Input: part model. Units: mm. Frame: model coordinates. A direction names the side the tool comes from. Round coordinates to 2 decimals unless told otherwise and drop trailing zeros. Order: outer loops, then holes, each group sorted by start corner. A loop starts at its lowest first (then second) coordinate and runs counter-clockwise, first axis right, second up. Notation, with made-up numbers: (-22, 43) - (1, 43) arc R6 cw to (1, 52) - close; hole circle Ø1 at (88, -16.5). An arc over 180 degrees is marked (long way). One line per item, written item: value. Start each with the question number.
from build123d import *

# Parameters (mm, degrees)
SKETCH1_W           = 31
SKETCH1_H           = 15
BOSS_EXTRUDE1_DEPTH = 6
SKETCH2_W           = 20.15
SKETCH2_H           = 6.15
CUT_EXTRUDE1_DEPTH  = 13
SKETCH6_R           = 5.45
SKETCH6_R_2         = 2.95
BOSS_EXTRUDE3_DEPTH = 3
CUT_EXTRUDE3_REACH  = 24.035
SKETCH3_W           = 1
SKETCH3_H           = 4
SKETCH3_W_2         = 2
SKETCH3_H_2         = 3.5
CUT_EXTRUDE4_START  = -3
SKETCH7_W           = 0.511909323
SKETCH7_H           = 0.870011062
SKETCH7_W_2         = 0.855337353
SKETCH7_H_2         = 1.408005392
CUT_EXTRUDE4_DEPTH  = 3
SKETCH8_W           = 31
SKETCH8_H           = 12
CUT_EXTRUDE5_DEPTH  = 3
CUT_EXTRUDE6_REACH  = 25.126
SKETCH9_R           = 1
SKETCH10_R          = 2.625
CUT_EXTRUDE7_DEPTH  = 2
SKETCH11_R          = 2.625
CUT_EXTRUDE8_DEPTH  = 2
CUT_EXTRUDE9_DEPTH  = 15
FILLET3_R           = 0.75
CUT_EXTRUDE10_DEPTH = 12
CHAMFER2_SIZE       = 1
FILLET4_R           = 0.75
CHAMFER3_SIZE       = 1.25
CUT_EXTRUDE11_DEPTH = 0.4


with BuildPart() as part:
    # Sketch1 → Boss-Extrude1 (new, symmetric)
    with BuildSketch(Plane.XY):
        Rectangle(SKETCH1_W, SKETCH1_H)
    extrude(amount=BOSS_EXTRUDE1_DEPTH, both=True)

    # Sketch2 → Cut-Extrude1 (cut)
    with BuildSketch(Plane.XZ.offset(7.5)):
        Rectangle(SKETCH2_W, SKETCH2_H)
    extrude(amount=-CUT_EXTRUDE1_DEPTH, mode=Mode.SUBTRACT)

    # Sketch6 → Boss-Extrude3 (add)
    # profile 1 of 2: a face of its own
    with BuildSketch(Plane(origin=(0, 7.5, 0), x_dir=(1, 0, 0), z_dir=(0, 1, 0))):
        with Locations(Location((-11.3, 0, 0), (0, 0, 140.41159309))):
            Circle(SKETCH6_R)
        with Locations(Location((-11.3, 0, 0), (0, 0, 270))):
            Circle(SKETCH6_R_2, mode=Mode.SUBTRACT)
    # profile 2 of 2: a face of its own
    with BuildSketch(Plane(origin=(0, 7.5, 0), x_dir=(1, 0, 0), z_dir=(0, 1, 0))):
        with Locations(Location((11.3, 0, 0), (0, 0, 39.58840691))):
            Circle(SKETCH6_R)
        with Locations(Location((11.3, 0, 0), (0, 0, 270))):
            Circle(SKETCH6_R_2, mode=Mode.SUBTRACT)
    extrude(amount=BOSS_EXTRUDE3_DEPTH)

    # Cut-Extrude3: up to this face of the body (flat: up to its plane)
    cut_extrude3_end = Plane(part.part.faces().sort_by_distance((-7.218793939, 10.5, 3.374876584))[0])
    # Sketch3 → Cut-Extrude3 (cut, up to the picked face)
    with BuildSketch(Plane.XZ.offset(-5.5), mode=Mode.PRIVATE) as cut_extrude3_sk1:
        with Locations((8.075, 0)):
            Rectangle(SKETCH3_W, SKETCH3_H)
    cut_extrude3_tool1 = split(extrude(cut_extrude3_sk1.sketch, amount=-CUT_EXTRUDE3_REACH, mode=Mode.PRIVATE), bisect_by=cut_extrude3_end, keep=Keep.BOTH, mode=Mode.PRIVATE)
    # Sketch3 → Cut-Extrude3 (cut, up to the picked face)
    with BuildSketch(Plane.XZ.offset(-5.5), mode=Mode.PRIVATE) as cut_extrude3_sk2:
        with Locations((-8.075, 0)):
            Rectangle(SKETCH3_W, SKETCH3_H)
    cut_extrude3_tool2 = split(extrude(cut_extrude3_sk2.sketch, amount=-CUT_EXTRUDE3_REACH, mode=Mode.PRIVATE), bisect_by=cut_extrude3_end, keep=Keep.BOTH, mode=Mode.PRIVATE)
    # Sketch3 → Cut-Extrude3 (cut, up to the picked face)
    with BuildSketch(Plane.XZ.offset(-5.5), mode=Mode.PRIVATE) as cut_extrude3_sk3:
        with Locations((-0.825, 0)):
            Rectangle(SKETCH3_W_2, SKETCH3_H_2)
    cut_extrude3_tool3 = split(extrude(cut_extrude3_sk3.sketch, amount=-CUT_EXTRUDE3_REACH, mode=Mode.PRIVATE), bisect_by=cut_extrude3_end, keep=Keep.BOTH, mode=Mode.PRIVATE)
    add(cut_extrude3_tool1.solids().sort_by(Axis((8.075, 5.5, 0), (0, 1, 0)))[0], mode=Mode.SUBTRACT)
    add(cut_extrude3_tool2.solids().sort_by(Axis((-8.075, 5.5, 0), (0, 1, 0)))[0], mode=Mode.SUBTRACT)
    add(cut_extrude3_tool3.solids().sort_by(Axis((-0.825, 5.5, 0), (0, 1, 0)))[0], mode=Mode.SUBTRACT)

    # Sketch7 → Cut-Extrude4 (cut)
    with BuildSketch(Plane(origin=(0, 10.5, 0), x_dir=(1, 0, 0), z_dir=(0, 1, 0)).offset(CUT_EXTRUDE4_START)):
        with BuildLine():
            ThreePointArc((-8.575, 1.129988938), (-8.814868985, 1.58953573), (-9.131475156, 2))
            Line((-9.131475156, 2), (-9.143163494, 2))
            Line((-9.143163494, 2), (-9.143163494, 0.699379733))
            Line((-9.143163494, 0.699379733), (-8.575, 0.699379733))
            Line((-8.575, 0.699379733), (-8.575, 1.129988938))
        make_face()
        with BuildLine():
            Line((-8.575, 1.129988938), (-8.575, 2))
            Line((-8.575, 2), (-9.131475156, 2))
            ThreePointArc((-9.131475156, 2), (-8.814868985, 1.58953573), (-8.575, 1.129988938))
        make_face()
        with BuildLine():
            ThreePointArc((-8.575, -1.129988938), (-8.814868985, -1.58953573), (-9.131475156, -2))
            Line((-9.131475156, -2), (-8.575, -2))
            Line((-8.575, -2), (-8.575, -1.129988938))
        make_face()
        with BuildLine():
            Line((-9.143163494, -2), (-9.131475156, -2))
            ThreePointArc((-9.131475156, -2), (-8.814868985, -1.58953573), (-8.575, -1.129988938))
            Line((-8.575, -1.129988938), (-8.575, -0.709964508))
            Line((-8.575, -0.709964508), (-9.143163494, -0.709964508))
            Line((-9.143163494, -0.709964508), (-9.143163494, -2))
        make_face()
        with Locations((8.830954662, 1.564994469)):
            Rectangle(SKETCH7_W, SKETCH7_H)
        with Locations((9.002668677, -1.295997304)):
            Rectangle(SKETCH7_W_2, SKETCH7_H_2)
    extrude(amount=CUT_EXTRUDE4_DEPTH, mode=Mode.SUBTRACT)

    # Sketch8 → Cut-Extrude5 (cut)
    with BuildSketch(Plane.XZ.offset(7.5)):
        Rectangle(SKETCH8_W, SKETCH8_H)
    extrude(amount=-CUT_EXTRUDE5_DEPTH, mode=Mode.SUBTRACT)

    # Cut-Extrude6: up to this face of the body (flat: up to its plane)
    cut_extrude6_end = Plane(part.part.faces().sort_by_distance((0, 1.5, -6))[0])
    # Sketch9 → Cut-Extrude6 (cut, up to the picked face)
    with BuildSketch(Plane.XY.offset(6), mode=Mode.PRIVATE) as cut_extrude6_sk1:
        with Locations((4.82, 1.5)):
            Circle(SKETCH9_R)
    cut_extrude6_tool1 = split(extrude(cut_extrude6_sk1.sketch, amount=-CUT_EXTRUDE6_REACH, mode=Mode.PRIVATE), bisect_by=cut_extrude6_end, keep=Keep.BOTH, mode=Mode.PRIVATE)
    # Sketch9 → Cut-Extrude6 (cut, up to the picked face)
    with BuildSketch(Plane.XY.offset(6), mode=Mode.PRIVATE) as cut_extrude6_sk2:
        with Locations((-4.82, 1.5)):
            Circle(SKETCH9_R)
    cut_extrude6_tool2 = split(extrude(cut_extrude6_sk2.sketch, amount=-CUT_EXTRUDE6_REACH, mode=Mode.PRIVATE), bisect_by=cut_extrude6_end, keep=Keep.BOTH, mode=Mode.PRIVATE)
    add(cut_extrude6_tool1.solids().sort_by(Axis((4.82, 1.5, 6), (0, 0, -1)))[0], mode=Mode.SUBTRACT)
    add(cut_extrude6_tool2.solids().sort_by(Axis((-4.82, 1.5, 6), (0, 0, -1)))[0], mode=Mode.SUBTRACT)

    # Sketch10 → Cut-Extrude7 (cut)
    with BuildSketch(Plane.XY.offset(6)):
        with Locations((4.82, 1.5)):
            Circle(SKETCH10_R)
    extrude(amount=-CUT_EXTRUDE7_DEPTH, mode=Mode.SUBTRACT)

    # Sketch11 → Cut-Extrude8 (cut)
    with BuildSketch(Plane(origin=(0, 0, -6), x_dir=(-1, 0, 0), z_dir=(0, 0, -1))):
        with Locations((4.82, 1.5)):
            Circle(SKETCH11_R)
    extrude(amount=-CUT_EXTRUDE8_DEPTH, mode=Mode.SUBTRACT)

    # Sketch12 → Cut-Extrude9 (cut)
    with BuildSketch(Plane.XZ.offset(4.5)):
        with BuildLine():
            Line((15.5, 3.473110997), (15.5, -3.473110997))
            ThreePointArc((15.5, -3.473110997), (16.75, 0), (15.5, 3.473110997))
        make_face()
        with BuildLine():
            Line((-15.5, -3.473110997), (-15.5, 3.473110997))
            ThreePointArc((-15.5, 3.473110997), (-16.75, 0), (-15.5, -3.473110997))
        make_face()
    extrude(amount=-CUT_EXTRUDE9_DEPTH, mode=Mode.SUBTRACT)

    # Fillet3
    fillet3_edges = [part.edges().sort_by_distance(p)[0] for p in [
        (-5.85, 10.5, 0),
        (5.85, 10.5, 0),
    ]]
    fillet(fillet3_edges, radius=FILLET3_R)

    # Sketch13 → Cut-Extrude10 (cut)
    with BuildSketch(Plane.XY.offset(6)):
        Polygon((13.5, -4.5), (11.5, 3.166935416), (15.5, 5), (15.5, -4.5), align=None)
        Polygon((-15.5, 5), (-15.5, -4.5), (-13.5, -4.5), (-11.5, 3.166935416), align=None)
    extrude(amount=-CUT_EXTRUDE10_DEPTH, mode=Mode.SUBTRACT)

    # Chamfer2
    chamfer2_edges = [part.edges().sort_by_distance(p)[0] for p in [
        (-15.5, 6.25, 6),
        (15.5, 6.25, -6),
        (15.5, 6.25, 6),
        (13.5, 4.083467708, 6),
        (12.5, -0.666532292, 6),
        (12.5, -0.666532292, -6),
        (13.5, 4.083467708, -6),
        (-13.5, 4.083467708, 6),
        (-12.5, -0.666532292, 6),
        (-13.5, 4.083467708, -6),
        (-12.5, -0.666532292, -6),
        (-15.5, 6.25, -6),
    ]]
    chamfer(chamfer2_edges, length=CHAMFER2_SIZE)

    # Fillet4
    fillet4_edges = [part.edges().sort_by_distance(p)[0] for p in [
        (15.5, 7.5, -4.236555499),
        (0, 7.5, 6),
        (-15.5, 7.5, 4.236555499),
        (15.5, 7.5, 4.236555499),
        (0, 7.5, -6),
        (-15, 7.5, 5.5),
        (-15, 7.5, -5.5),
        (15, 7.5, -5.5),
        (15, 7.5, 5.5),
        (-15.5, 7.5, -4.236555499),
    ]]
    fillet(fillet4_edges, radius=FILLET4_R)

    # Chamfer3
    chamfer3_edges = [part.edges().sort_by_distance(p)[0] for p in [
        (0, -4.5, 3.075),
        (10.075, -4.5, 0),
        (0, -4.5, -3.075),
        (-10.075, -4.5, 0),
    ]]
    chamfer(chamfer3_edges, length=CHAMFER3_SIZE)

    # Sketch14 → Cut-Extrude11 (cut)
    with BuildSketch(Plane(origin=(15.5, 0, 0), x_dir=(0, 0, -1), z_dir=(1, 0, 0))):
        Polygon((-1, 6), (1, 6), (1, 8.5), (1.5, 8.5), (0, 10), (-1.5, 8.5), (-1, 8.5), align=None)
    extrude(amount=-CUT_EXTRUDE11_DEPTH, mode=Mode.SUBTRACT)


solid = part.part
1. Set-up query: faces 5 (the face through (-14, 7.5, -5)), 6 (the face through (-14, 7.5, 5)), 7 (the face through (14.25, 8.98, 0.07)). Return all of +Z, -Z, +X, -X, +Y, -Y with unobstructed straight access to the full face (end or side cutting, diameter ignored); none if empty.
2. Line query: line 1 (Z direction, x = 3, y = 4) (3 decimals); line 2 (X direction, y = 9, z = -2.25); line 3 (X direction, y = 9.25, z = -2.5). Output: solid intervals per line, ascending. Write a range as from..to.
3. Section A-A (x = -4.82). Return the cut outline in (y, z) (3 decimals), then the cut area to 3 significant figures.
4. Pull-direction query (Z, two-part tool) for faces 1 (the face through (-14.834, 7.286, 5.348)), 2 (the face through (-8.575, 6, 0)), 3 (the face through (5.28, 0.61, -4.52)), 4 (the face through (5.853, 8.562, -0.187)); classes: released by +Z, released by -Z, zero draft, split by the parting line, or undercut.
5. Pin query (flat end, axial travel): pin 1 (2 mm diameter, centred on x = -4, y = 8, fed in from +Z); pin 2 (0.5 mm diameter, centred on x = 14, z = -4.5, fed in from +Y); pin 3 (4 mm diameter, centred on x = 4.5, y = 1, fed in from +Z). Return the tip coordinate at first contact, or that it passes through.
6. Section B-B (z = 0.5). State how many separate pieces and enclosed holes the cut face has, then the cut area to 3 significant figures.
Solved:
1. face 5: -Z, -X, +Y
1. face 6: +Z, -X, +Y
1. face 7: +Y
2. line 1: z = -6..-3.075, 3.075..6
2. line 2: x = -15.5..-13.21, -9.39..-6.34, 6.34..9.39, 13.21..15.5
2. line 3: x = -15.5..-12.87, -9.73..-6.46, 6.46..9.73, 12.87..15.5
3. outline: (-4.5, -6) - (-1.125, -6) - (-1.125, -4) - (0.5, -4) - (0.5, -3.075) - (-3.25, -3.075) - (-4.5, -4.325) - close; (-4.5, 4.325) - (-3.25, 3.075) - (0.5, 3.075) - (0.5, 6) - (-4.5, 6) - close; (2.5, -4) - (4.125, -4) - (4.125, -6) - (6.75, -6) arc R0.75 ccw to (7.5, -5.25) - (7.5, 5.25) arc R0.75 ccw to (6.75, 6) - (2.5, 6) - (2.5, 3.075) - (5.5, 3.075) - (5.5, -3.075) - (2.5, -3.075) - close
3. area: 62.5 mm²
4. face 1: released by +Z
4. face 2: undercut
4. face 3: zero draft
4. face 4: split by the parting line
5. pin 1: stops at z = 5.96
5. pin 2: stops at y = 10.44
5. pin 3: stops at z = 4
6. separate pieces: 4
6. enclosed holes: 0
6. area: 124 mm²
